Answer from the drawing. Dimensions are ordinates in mm from the lowest x, y and z of the part. Give positions to 0.01 mm unless a question says otherwise; leave off trailing zeros. Write each loop counter-clockwise with the first axis right and the second up, starting at its lowest first coordinate (ties: lowest second). Pieces come first, ordered by that corner, then holes. Notation, with made-up numbers: (43, 64) - (75, 64) arc R17 ccw to (75, 87) - close; hole circle Ø10 at (45.25, -6). An arc over 180 degrees is marked (long way). Answer as a JSON object with one key per item and string values. Group by question number.
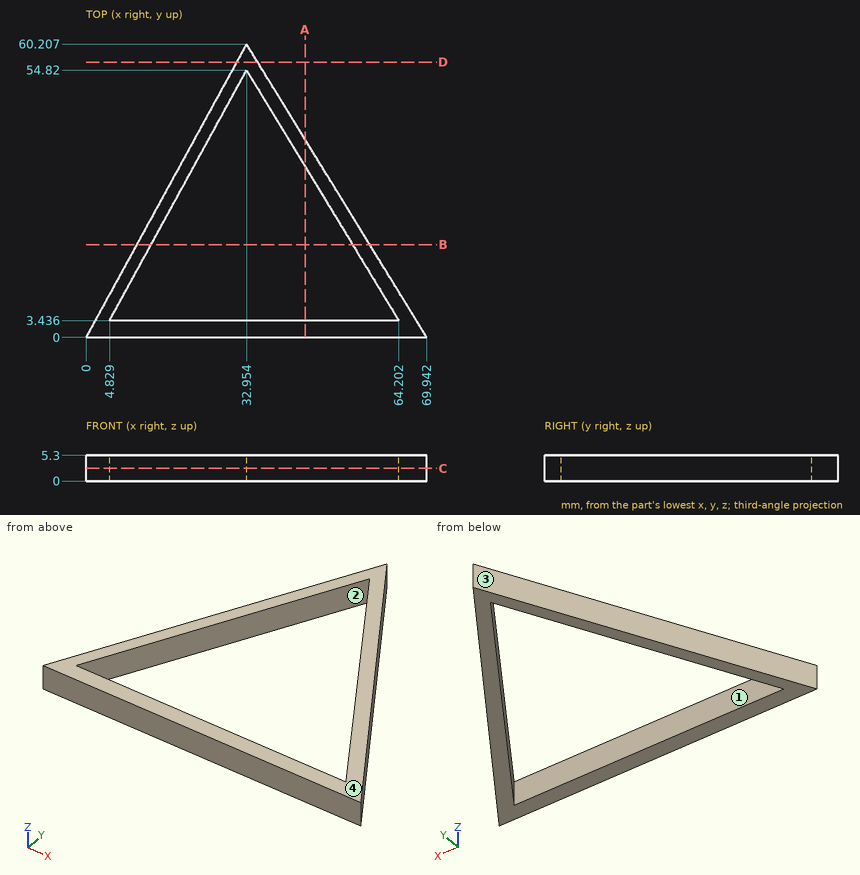
1) Flat-ended cylindrical pins translate along their axes: pin 1 Ø1.5 at (y, z) = (29, 3) entering from +X; pin 2 Ø1.5 at (y, z) = (45.5, 3) entering from -X (1 decimal); pin 3 Ø1.6 at (x, z) = (34, 3.5) entering from +Y (1 decimal). Find the tip coordinate at first contact, or state that the pin passes through.
2) For a pull along Y with two mould halves and no side action, classify the marked faces 1, 2, 3 and 4 as released by +Y, released by -Y, zero draft, split by the parting line, or undercut.
3) Find section A-A, the plane x = 45. Write down the section's boundary in (y, z).
4) Find section B-B, the plane y = 19. Write down the section's boundary in (x, z).
5) Find section D-D, the plane y = 56.5. Write down the section's boundary in (x, z) (1 decimal).
6) Find the intervals of material crossed by line 1 (X direction, y = 8.5, z = 1.65); line 2 (X direction, y = 16, z = 2.1) (1 decimal); line 3 (Y direction, x = 25, z = 2.5) (1 decimal), in increasing order. Write a range as [from, to].
7) Find section C-C, the plane z = 2.6. Write down the section's boundary in (x, y) (1 decimal).
Values follow:
{
 "1": {"pin 1": "stops at x = 52.59", "pin 2": "stops at x = 24.5", "pin 3": "stops at y = 59.8"},
 "2": {"face 1": "undercut", "face 2": "undercut", "face 3": "released by +Y", "face 4": "zero draft"},
 "3": {"outline": "(0, 0) - (3.44, 0) - (3.44, 5.3) - (0, 5.3) - close; (35.01, 0) - (40.6, 0) - (40.6, 5.3) - (35.01, 5.3) - close"},
 "4": {"outline": "(10.4, 0) - (13.35, 0) - (13.35, 5.3) - (10.4, 5.3) - close; (54.74, 0) - (58.27, 0) - (58.27, 5.3) - (54.74, 5.3) - close"},
 "5": {"outline": "(30.9, 0) - (35.2, 0) - (35.2, 5.3) - (30.9, 5.3) - close"},
 "6": {"line 1": "x = [4.65, 7.6], [61.12, 64.72]", "line 2": "x = [8.8, 11.7], [56.6, 60.1]", "line 3": "y = [0, 3.4], [40.3, 45.7]"},
 "7": {"outline": "(0, 0) - (69.9, 0) - (33, 60.2) - close; hole (4.8, 3.4) - (64.2, 3.4) - (33, 54.8) - close"}
}
